Part model, mm, in its own coordinate system. Face numbers are marked on the shaded views. A direction names the side the tool comes from. Round coordinates to 2 decimals unless told otherwise and drop trailing zeros. Order: outer loops, then holes, each group sorted by start corner. A loop starts at its lowest first (then second) coordinate and runs counter-clockwise, first axis right, second up. Notation, with made-up numbers: M 73.5,56 L 80.5,56 A31 cw 80.5,88 Z; hole C -8.75,36.25 d1. An arc over 180 degrees is marked long. Write each question's results on one line, items separated by ' | '. Start each with the question number.
1. Band-saw the part on C-C, the plane z = 2. List the corners of the cut face in (x, y).
2. Two-plate mould, pull along Y, no slides. Class the marked faces 3, 4 and 5: +Y half, -Y half, draft (parallel to the pull), parting line (faces both ways), or undercut.
3. Band-saw the part on A-A, the plane y = 3. List the corners of the cut face in (x, z).
4. Which spindle directions (+Z, -Z, +X, -X, +Y, -Y) get a long thin tool onto all of the face, cutting with end or side? Do the marked faces 1 and 2. Say none if no direction does.
5. Probe L1, parallel to X at y = 4.5, z = 1.5; L2, parallel to X at y = 7.75, z = 2.75; L3, parallel to Y at x = 2.25, z = 5.75. List the from-to ranges inside material, lowest first. Write a range as [from, to].
6. Band-saw the part on B-B, the plane x = 3. List the corners of the cut face in (y, z), then the cut area to 3 significant figures.
7. Band-saw the part on D-D, the plane x = -3.5. List the corners of the cut face in (y, z).
```python
from build123d import *

# Parameters (mm, degrees)
BOSS_EXTRUDE1_DEPTH = 10
SKETCH2_W           = 11.202256629
SKETCH2_H           = 10
BOSS_EXTRUDE2_DEPTH = 4


with BuildPart() as part:
    # Sketch1 → Boss-Extrude1 (new body)
    with BuildSketch(Plane.XY):
        with BuildLine():
            Line((-4.000846014, 2.113625207), (-6.3997177, 2.113625207))
            Line((-6.3997177, 2.113625207), (-6.3997177, 13.316105715))
            Line((-6.3997177, 13.316105715), (4.802538929, 13.316105715))
            Line((4.802538929, 13.316105715), (4.802538929, 2.113625207))
            Line((4.802538929, 2.113625207), (2.403667244, 2.113625207))
            Line((2.403667244, 2.113625207), (2.403667244, 4.919117505))
            ThreePointArc((2.403667244, 4.919117505), (-0.798589385, 11.316105715), (-4.000846014, 4.919117505))
            Line((-4.000846014, 4.919117505), (-4.000846014, 2.113625207))
        make_face()
    extrude(amount=BOSS_EXTRUDE1_DEPTH)

    # Sketch2 → Boss-Extrude2 (add)
    with BuildSketch(Plane(origin=(0, 13.316105715, 0), x_dir=(1, 0, 0), z_dir=(0, 1, 0))):
        with Locations((-0.798589385, -5)):
            Rectangle(SKETCH2_W, SKETCH2_H)
    extrude(amount=BOSS_EXTRUDE2_DEPTH)


solid = part.part
```
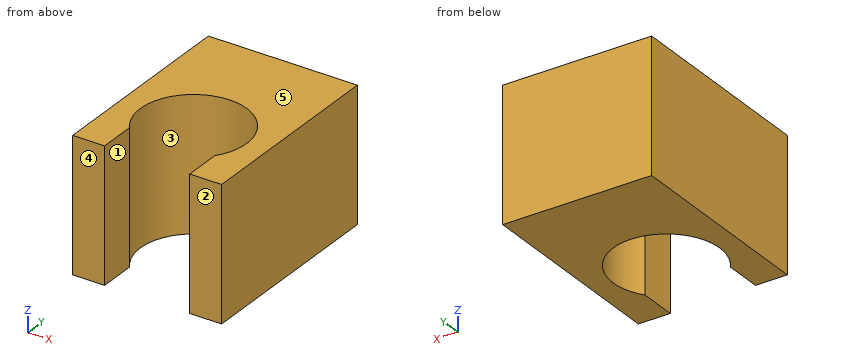
Solution:
1) outline: M -6.4,2.11 L -4,2.11 L -4,4.92 A4 cw long 2.4,4.92 L 2.4,2.11 L 4.8,2.11 L 4.8,17.32 L -6.4,17.32 Z
2) face 3: undercut | face 4: -Y half | face 5: draft
3) outline: M -6.4,0 L -4,0 L -4,10 L -6.4,10 Z; M 2.4,0 L 4.8,0 L 4.8,10 L 2.4,10 Z
4) face 1: +Z, -Z, -Y | face 2: +Z, -Z, +X, -X, -Y
5) L1: [-6.4, -4], [2.4, 4.8] | L2: [-6.4, -4.77], [3.18, 4.8] | L3: [9.91, 17.32]
6) outline: M 2.11,0 L 6.06,0 L 6.06,10 L 2.11,10 Z; M 8.57,0 L 17.32,0 L 17.32,10 L 8.57,10 Z | area: 127 mm^2
7) outline: M 10.27,0 L 17.32,0 L 17.32,10 L 10.27,10 Z
